from build123d import *

# Parameters (mm, degrees)
SKETCH1_W                  = 254
SKETCH1_H                  = 31.75
BOSS_EXTRUDE1_DEPTH        = 25.4
BOSS_EXTRUDE1_DEPTH_BACK   = 25.4
SKETCH1_R                  = 9.525
BOSS_EXTRUDE1_2_DEPTH      = 25.4
BOSS_EXTRUDE1_2_DEPTH_BACK = 25.4
BOSS_EXTRUDE1_3_DEPTH      = 25.4
BOSS_EXTRUDE1_3_DEPTH_BACK = 25.4
BOSS_EXTRUDE2_START        = 25.4
SKETCH1_4_R                = 15.875
SKETCH1_4_R_2              = 9.525
BOSS_EXTRUDE2_DEPTH        = 9.525
BOSS_EXTRUDE3_START        = -25.4
SKETCH1_5_R                = 15.875
SKETCH1_5_R_2              = 9.525
BOSS_EXTRUDE3_DEPTH        = 9.525


with BuildPart() as part:
    # Sketch1 → Boss-Extrude1 (new body, two sides)
    with BuildSketch(Plane.XY) as boss_extrude1_sk:
        Rectangle(SKETCH1_W, SKETCH1_H)
    extrude(amount=BOSS_EXTRUDE1_DEPTH)
    extrude(boss_extrude1_sk.sketch, amount=-BOSS_EXTRUDE1_DEPTH_BACK)



with BuildPart() as body_2:
    # Sketch1 → Boss-Extrude1 2 (new body, two sides)
    with BuildSketch(Plane.XY) as boss_extrude1_2_sk:
        with Locations((-142.875, 0)):
            Circle(SKETCH1_R)
    extrude(amount=BOSS_EXTRUDE1_2_DEPTH)
    extrude(boss_extrude1_2_sk.sketch, amount=-BOSS_EXTRUDE1_2_DEPTH_BACK)


with BuildPart() as body_3:
    # Sketch1 → Boss-Extrude1 3 (new body, two sides)
    with BuildSketch(Plane.XY) as boss_extrude1_3_sk:
        with Locations((142.875, 0)):
            Circle(SKETCH1_R)
    extrude(amount=BOSS_EXTRUDE1_3_DEPTH)
    extrude(boss_extrude1_3_sk.sketch, amount=-BOSS_EXTRUDE1_3_DEPTH_BACK)


with BuildPart() as part_1:
    add(part.part)

    add(body_2.part)  # Boss-Extrude2 merges body 2

    add(body_3.part)  # Boss-Extrude2 merges body 3
    # Sketch1<4> → Boss-Extrude2 (add)
    with BuildSketch(Plane.XY.offset(BOSS_EXTRUDE2_START)):
        with BuildLine():
            Line((-127, 15.875), (-142.875, 15.875))
            ThreePointArc((-142.875, 15.875), (-131.649679849, 11.225320151), (-127, 0))
            Line((-127, 0), (-127, 15.875))
        make_face()
        with Locations((-142.875, 0)):
            Circle(SKETCH1_4_R)
        with Locations((-142.875, 0)):
            Circle(SKETCH1_4_R_2, mode=Mode.SUBTRACT)
        with BuildLine():
            Line((-127, -15.875), (-127, 0))
            ThreePointArc((-127, 0), (-131.649679849, -11.225320151), (-142.875, -15.875))
            Line((-142.875, -15.875), (-127, -15.875))
        make_face()
        with BuildLine():
            Line((142.875, 15.875), (127, 15.875))
            Line((127, 15.875), (127, 3.4e-08))
            ThreePointArc((127, 3.4e-08), (131.649679861, 11.225320163), (142.875, 15.875))
        make_face()
        with Locations((142.875, 0)):
            Circle(SKETCH1_4_R)
        with Locations((142.875, 0)):
            Circle(SKETCH1_4_R_2, mode=Mode.SUBTRACT)
        with BuildLine():
            ThreePointArc((142.875, -15.875), (131.649679837, -11.225320139), (127, 3.4e-08))
            Line((127, 3.4e-08), (127, -15.875))
            Line((127, -15.875), (142.875, -15.875))
        make_face()
    extrude(amount=-BOSS_EXTRUDE2_DEPTH)

    # Sketch1<5> → Boss-Extrude3 (add)
    with BuildSketch(Plane.XY.offset(BOSS_EXTRUDE3_START)):
        with Locations((-142.875, 0)):
            Circle(SKETCH1_5_R)
        with Locations((-142.875, 0)):
            Circle(SKETCH1_5_R_2, mode=Mode.SUBTRACT)
        with BuildLine():
            Line((-127, 15.875), (-142.875, 15.875))
            ThreePointArc((-142.875, 15.875), (-131.649679849, 11.225320151), (-127, 0))
            Line((-127, 0), (-127, 15.875))
        make_face()
        with BuildLine():
            Line((-127, -15.875), (-127, 0))
            ThreePointArc((-127, 0), (-131.649679849, -11.225320151), (-142.875, -15.875))
            Line((-142.875, -15.875), (-127, -15.875))
        make_face()
        with BuildLine():
            Line((142.875, 15.875), (127, 15.875))
            Line((127, 15.875), (127, 3.4e-08))
            ThreePointArc((127, 3.4e-08), (131.649679861, 11.225320163), (142.875, 15.875))
        make_face()
        with Locations((142.875, 0)):
            Circle(SKETCH1_5_R)
        with Locations((142.875, 0)):
            Circle(SKETCH1_5_R_2, mode=Mode.SUBTRACT)
        with BuildLine():
            ThreePointArc((142.875, -15.875), (131.649679837, -11.225320139), (127, 3.4e-08))
            Line((127, 3.4e-08), (127, -15.875))
            Line((127, -15.875), (142.875, -15.875))
        make_face()
    extrude(amount=BOSS_EXTRUDE3_DEPTH)


solid = part_1.part
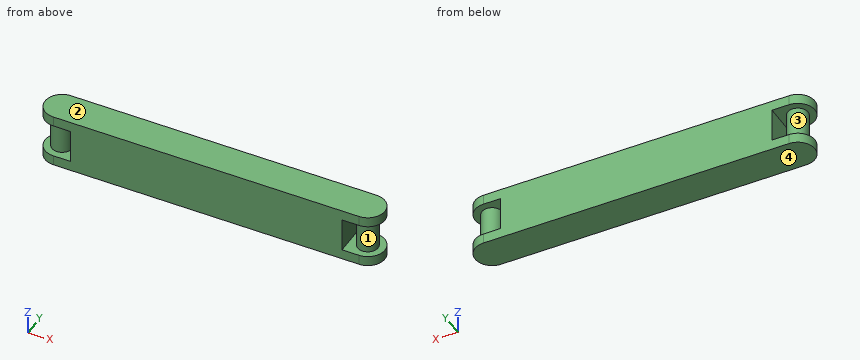
Can you work these out from the model? Positions are in its coordinate system, mm. Face numbers are marked on the shaded views. A direction names the side the tool comes from. Give positions to 0.01 mm unless a question says otherwise; leave off trailing zeros. Order: outer loops, then holes, each group sorted by start corner. A loop starts at its lowest first (then second) coordinate and runs counter-clockwise, first axis right, second up. Notation, with made-up numbers: M -33.75,-19 L 1.25,-19 A24 cw 1.25,-2 Z; hole C 64.25,50.5 d11. An arc over 180 degrees is marked long. Use one line per item in the form item = value. Start each with the question number.
Item 1: If we section it at C-C (z = -22): Write out the boundary of the cut face in (x, y) (3 decimals).
Item 2: If we section it at B-B (y = 0): Write out the boundary of the cut face in (x, z) (3 decimals).
Item 3: If I drill on line 1 along X through (y, z) = (0.5, 8); line 2 along X through (y, z) = (-4.5, 7); line 3 along X through (y, z) = (14.5, -9), over which ranges is the centre line in solid material (lowest first)?
Item 4: If we section it at A-A (z = -4): Write out the boundary of the cut face in (x, y) (3 decimals), then the cut area to 3 significant figures.
Item 5: For the marked faces 3 and 4, which set-ups out of +Z, -Z, +X, -X, +Y, -Y let a thin tool reach every point of the face, with its end or its side?
Item 6: We'd pull the mould along X, two halves only. Please class the marked faces 1 and 2: +X half, -X half, draft (parallel to the pull), parting line (faces both ways), or undercut.
Item 7: Will these pins go through, and if not, where does the flat tip stop? pin 1 Ø5 at (y, z) = (7.5, 12.5) entering from -X; pin 2 Ø6 at (y, z) = (-7.5, 1.5) entering from -X; pin 3 Ø1 at (y, z) = (10, 16) entering from -X.
Outcome:
q1.outline = M -142.875,-15.875 L 142.875,-15.875 A15.875 ccw 142.875,15.875 L -142.875,15.875 A15.875 ccw Z
q2.outline = M -158.75,-25.4 L 158.75,-25.4 L 158.75,-15.875 L 152.4,-15.875 L 152.4,15.875 L 158.75,15.875 L 158.75,25.4 L -158.75,25.4 L -158.75,15.875 L -152.4,15.875 L -152.4,-15.875 L -158.75,-15.875 Z; hole M -133.35,-15.875 L -127,-15.875 L -127,15.875 L -133.35,15.875 Z; hole M 127,-15.875 L 133.35,-15.875 L 133.35,15.875 L 127,15.875 Z
q3.line_1 = -152.39 to -133.36, -127 to 127, 133.36 to 152.39
q3.line_2 = -151.27 to -134.48, -127 to 127, 134.48 to 151.27
q3.line_3 = -127 to 127
q4.outline = C -142.875,0 d19.05; M -127,-15.875 L 127,-15.875 L 127,15.875 L -127,15.875 Z; C 142.875,0 d19.05
q4.area = 8,630 mm2
q5.face_3 = none
q5.face_4 = -Z, +X, -X, +Y, -Y
q6.face_1 = undercut
q6.face_2 = draft
q7.pin_1 = -150.98
q7.pin_2 = -151.27
q7.pin_3 = -155.59
